```python
from build123d import *

# Parameters (mm, degrees)
BOSS_EXTRUDE1_DEPTH = 3


with BuildPart() as part:
    # Sketch1 → Boss-Extrude1 (new body)
    with BuildSketch(Plane(origin=(0, 0, 0), x_dir=(1, 0, 0), z_dir=(0, 0, -1))):
        Polygon((40, 0), (55, 0), (55, -3), (75, -3), (75, 0), (90, 0), (90, -3), (110, -3), (110, 0), (125, 0), (125, -3), (145, -3), (145, 0), (160, 0), (160, -3), (180, -3), (180, 0), (200, 0), (200, 35), (180, 35), (180, 32), (160, 32), (160, 35), (145, 35), (145, 32), (125, 32), (125, 35), (110, 35), (110, 32), (90, 32), (90, 35), (75, 35), (75, 32), (55, 32), (55, 35), (40, 35), (40, 32), (20, 32), (20, 35), (0, 35), (0, 0), (20, 0), (20, -3), (40, -3), align=None)
    extrude(amount=BOSS_EXTRUDE1_DEPTH)


solid = part.part
```
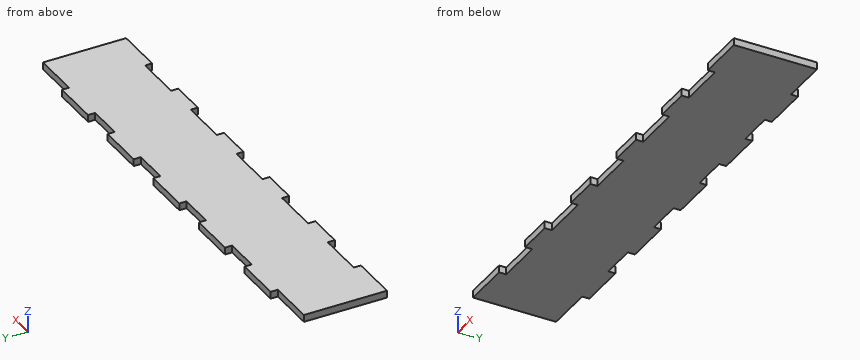
Check sheet for the modelled part. Datum: model origin and axes. Units: mm. Coordinates: 2 decimals unless noted, no trailing zeros. Order: outer loops, then holes, each group sorted by start corner. A loop starts at its lowest first (then second) coordinate and runs counter-clockwise, first axis right, second up. Notation, with made-up numbers: M 10.25,44.5 L 52.25,44.5 A13 cw 52.25,61.5 Z; hole C -8.75,27.25 d5. An arc over 180 degrees is marked long. One line per question, with ' | ' between items. Start each with the question number.
Item 1: Material ranges on line 1 (Y direction, x = 47, z = -0.3); line 2 (Y direction, x = 109, z = -1.4), recorded low to high.
Item 2: Gauge pin test, flat ends, axial feed: P1, Ø1, axis at y = -29, z = -2.5, coming from the -X side; P2, Ø1.5, axis at y = 2, z = -1.5, coming from the -X side; P3, Ø0.9, axis at x = 149.5, z = -1, coming from the +Y side; P4, Ø0.9, axis at y = 2, z = -2, coming from the +X side. Record the tip position at first contact, or that the pin passes through.
Item 3: Sectioned sample at A-A on x = 65.5. Record the cut outline in (y, z), and give its area (3 significant figures).
Answer below:
1) line 1: y = -35 to 0 | line 2: y = -32 to 3
2) P1: stops at x = 0 | P2: stops at x = 20 | P3: stops at y = 0 | P4: stops at x = 180
3) outline: M -32,-3 L 3,-3 L 3,0 L -32,0 Z | area: 105 mm^2
